Design review of the part shown in the three views and the two pictorial views. Dimensions are in mm from the part's minimum x, y and z. A direction names the side the tool comes from. Coordinates: 2 decimals unless noted, no trailing zeros. Loops run counter-clockwise (first coordinate to the right, second up) from the corner with the lowest first, then second, coordinate; pieces in that order, holes last. Notation, with made-up numbers: M 5,-33 L 32,-33 A6 ccw 32,-24 Z; hole C 31,-11.75 d6. An arc over 180 degrees is marked long. Use one line per item in the form item = value.
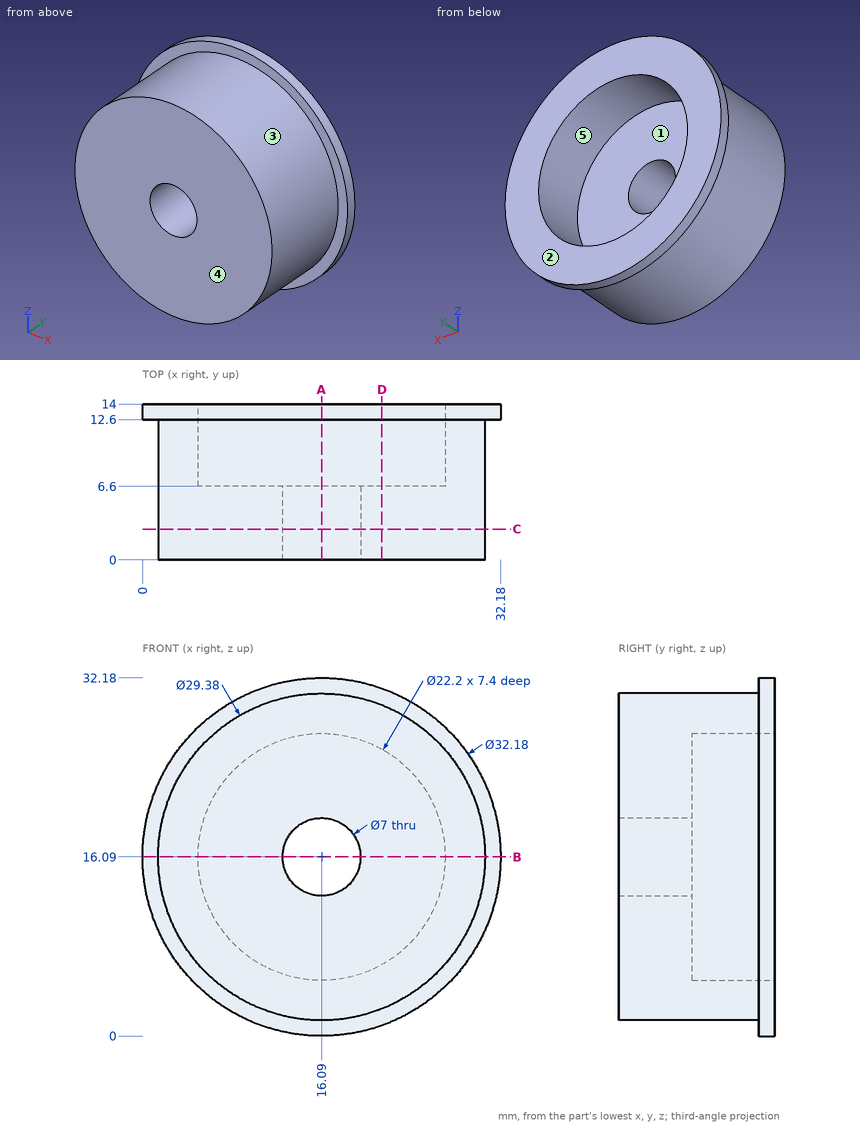
1. Wall thickness on line 1 along X through (y, z) = (11.5, 16.09); line 2 along X through (y, z) = (1.75, 16.09): over which ranges is each line inside the solid? List them lowest first. Write a range as from..to.
Response values:
line_1 = 1.4..4.99, 27.19..30.78
line_2 = 1.4..12.59, 19.59..30.78
2. Add section A-A (x = 16.09). State the section outline as (y, z) points.
Response values:
outline = M 0,1.4 L 12.6,1.4 L 12.6,0 L 14,0 L 14,4.99 L 6.6,4.99 L 6.6,12.59 L 0,12.59 Z; M 0,19.59 L 6.6,19.59 L 6.6,27.19 L 14,27.19 L 14,32.18 L 12.6,32.18 L 12.6,30.78 L 0,30.78 Z
3. Insertion check: P1, Ø1.5, axis at y = 2.5, z = 25.5, coming from the -X side; P2, Ø3, axis at x = 20, y = 3.5, coming from the -Z side; P3, Ø6.5, axis at x = 16.09, z = 16.09, coming from the +Y side; P4, Ø1, axis at y = 10.5, z = 11, coming from the +X side. Each pin has a flat end and moves straight along its axis. Give the tip position at first contact, or say it passes through.
Response values:
P1 = 4.22
P2 = 1.6
P3 = through
P4 = 30.04
4. Add section B-B (z = 16.09). State the section outline as (x, y) points, then the cut area to 3 significant figures.
Response values:
outline = M 0,12.6 L 1.4,12.6 L 1.4,0 L 12.59,0 L 12.59,6.6 L 4.99,6.6 L 4.99,14 L 0,14 Z; M 19.59,0 L 30.78,0 L 30.78,12.6 L 32.18,12.6 L 32.18,14 L 27.19,14 L 27.19,6.6 L 19.59,6.6 Z
area = 205 mm^2
5. Machinability: for the marked faces 1 and 2, which of the approach directions +Z, -Z, +X, -X, +Y, -Y give a long, thin tool a straight path to every point of the face, cutting with its end or side? Answer none if there is none.
Response values:
face_1 = +Y
face_2 = +Z, -Z, +X, -X, +Y
6. The part is to be moulded in two halves that separate along Z. For the marked faces 3, 4 and 5, say which applies: pulls with the +Z half, pulls with the -Z half, needs draft (parallel to the pull), parting line crosses it, or undercut.
Response values:
face_3 = parting line crosses it
face_4 = needs draft
face_5 = undercut
7. Add section C-C (y = 2.75). State the section outline as (x, z) points.
Response values:
outline = C 16.09,16.09 d29.38; hole C 16.09,16.09 d7
8. Add section D-D (x = 21.5). State the section outline as (y, z) points.
Response values:
outline = M 0,2.43 L 12.6,2.43 L 12.6,0.94 L 14,0.94 L 14,6.4 L 6.6,6.4 L 6.6,25.78 L 14,25.78 L 14,31.24 L 12.6,31.24 L 12.6,29.75 L 0,29.75 Z
